Read the model definition and answer for the solid it produces. Units are mm, in the model's axes. Face numbers are marked on the shaded views. A direction names the side the tool comes from. Give positions to 0.01 mm unless a question says otherwise; leave off trailing zeros. Loops run counter-clockwise (first coordinate to the right, second up) from the corner with the lowest first, then second, coordinate; pieces in that order, holes last. Notation, with made-up numbers: (63.5, 23.25) - (113.5, 23.25) arc R26 ccw to (113.5, 43.25) - close; hole circle Ø1 at (45, -32). An arc over 180 degrees is marked (long way). Write item = value, one per line.
```python
from build123d import *

# Parameters (mm, degrees)
SKETCH1_R           = 2
BOSS_EXTRUDE1_DEPTH = 19
SKETCH3_R           = 2
CUT_EXTRUDE2_DEPTH  = 40.953097502
SKETCH4_R           = 4
CUT_EXTRUDE3_DEPTH  = 1.5
CUT_EXTRUDE4_START  = -1.5
SKETCH5_R           = 4
CUT_EXTRUDE4_DEPTH  = 1.5


with BuildPart() as part:
    # Sketch1 → Boss-Extrude1 (new body)
    with BuildSketch(Plane.XY):
        with BuildLine():
            Line((-12.5, -13.5), (12.5, -13.5))
            ThreePointArc((12.5, -13.5), (19.571067812, -10.571067812), (22.5, -3.5))
            Line((22.5, -3.5), (22.5, 3.5))
            ThreePointArc((22.5, 3.5), (19.571067812, 10.571067812), (12.5, 13.5))
            Line((12.5, 13.5), (-12.5, 13.5))
            ThreePointArc((-12.5, 13.5), (-19.571067812, 10.571067812), (-22.5, 3.5))
            Line((-22.5, 3.5), (-22.5, -3.5))
            ThreePointArc((-22.5, -3.5), (-19.571067812, -10.571067812), (-12.5, -13.5))
        make_face()
        with Locations((-18, 0)):
            Circle(SKETCH1_R, mode=Mode.SUBTRACT)
        with Locations((18, 0)):
            Circle(SKETCH1_R, mode=Mode.SUBTRACT)
        with BuildLine():
            Line((-8, -10), (8, -10))
            ThreePointArc((8, -10), (9.414213562, -9.414213562), (10, -8))
            Line((10, -8), (10, 8))
            ThreePointArc((10, 8), (9.414213562, 9.414213562), (8, 10))
            Line((8, 10), (-8, 10))
            ThreePointArc((-8, 10), (-9.414213562, 9.414213562), (-10, 8))
            Line((-10, 8), (-10, -8))
            ThreePointArc((-10, -8), (-9.414213562, -9.414213562), (-8, -10))
        make_face(mode=Mode.SUBTRACT)
    extrude(amount=BOSS_EXTRUDE1_DEPTH)

    # Sketch3 → Cut-Extrude2 (cut, through all)
    with BuildSketch(Plane(origin=(0, 13.5, 0), x_dir=(1, 0, 0), z_dir=(0, 1, 0))):
        with Locations(Location((0, -9.5, 0), (0, 0, 270))):
            Circle(SKETCH3_R)
    extrude(amount=-CUT_EXTRUDE2_DEPTH, mode=Mode.SUBTRACT)

    # Sketch4 → Cut-Extrude3 (cut)
    with BuildSketch(Plane(origin=(0, 13.5, 0), x_dir=(1, 0, 0), z_dir=(0, 1, 0))):
        with Locations(Location((0, -9.5, 0), (0, 0, 270))):
            Circle(SKETCH4_R)
    extrude(amount=-CUT_EXTRUDE3_DEPTH, mode=Mode.SUBTRACT)

    # Sketch5 → Cut-Extrude4 (cut)
    with BuildSketch(Plane.XZ.offset(13.5).offset(CUT_EXTRUDE4_START)):
        with Locations(Location((0, 9.5, 0), (0, 0, 90))):
            Circle(SKETCH5_R)
    extrude(amount=CUT_EXTRUDE4_DEPTH, mode=Mode.SUBTRACT)


solid = part.part
```
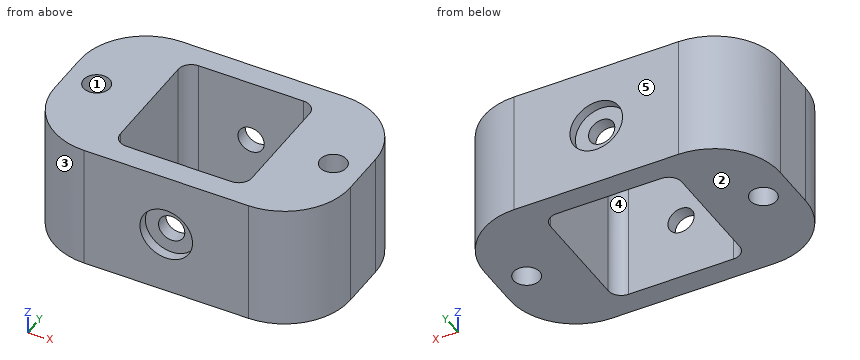
1) A tool of negligible diameter and unlimited length cuts with its end or side. For the marked faces 4 and 5, from which of +Z, -Z, +X, -X, +Y, -Y can it reach the whole face along a straight path? Write none if from no direction.
Output:
face_4 = +Z, -Z
face_5 = +Z, -Z, +X, -X, +Y
2) Each of these flat-tipped pins is pushed along its axis until it touches: P1, Ø2.5, axis at x = 0, z = 8, coming from the +Y side; P2, Ø7, axis at x = 0, z = 9.5, coming from the -Y side; P3, Ø3, axis at x = -16.5, z = 15, coming from the +Y side; P4, Ø2.5, axis at x = 18, y = 0, coming from the +Z side. Where does it stop, or does it pass through?
Output:
P1 = 12
P2 = -12
P3 = 13.18
P4 = through
3) A cutting plane is placed at C-C on x = -7. Determine the outline of the cut face in (y, z).
Output:
outline = (-13.5, 0) - (-10, 0) - (-10, 19) - (-13.5, 19) - close; (10, 0) - (13.5, 0) - (13.5, 19) - (10, 19) - close
4) A cutting plane is placed at B-B on x = 0. Determine the outline of the cut face in (y, z), then the cut area to 3 significant figures.
Output:
outline = (-13.5, 0) - (-10, 0) - (-10, 7.5) - (-12, 7.5) - (-12, 5.5) - (-13.5, 5.5) - close; (-13.5, 13.5) - (-12, 13.5) - (-12, 11.5) - (-10, 11.5) - (-10, 19) - (-13.5, 19) - close; (10, 0) - (13.5, 0) - (13.5, 5.5) - (12, 5.5) - (12, 7.5) - (10, 7.5) - close; (10, 11.5) - (12, 11.5) - (12, 13.5) - (13.5, 13.5) - (13.5, 19) - (10, 19) - close
area = 93.0 mm²
5) Find the intervals of material crossed by probe 1 along Y at (x, z) = (3.5, 5); probe 2 along X at (y, z) = (-2.25, 1); probe 3 along X at (y, z) = (-1.75, 4.25), in increasing order.
Output:
probe_1 = -13.5 to -10, 10 to 13.5
probe_2 = -22.5 to -10, 10 to 22.5
probe_3 = -22.5 to -18.97, -17.03 to -10, 10 to 17.03, 18.97 to 22.5
6) A cutting plane is placed at A-A on z = 9.5. Give the number of separate pieces and of enclosed holes in the cut face, then the cut area to 3 significant figures.
Output:
separate_pieces = 2
enclosed_holes = 2
area = 667 mm²
7) The mould has two halves that part along Y. Classify the marked faces 1, 2 and 3: pulls with the +Y half, pulls with the -Y half, needs draft (parallel to the pull), parting line crosses it, or undercut.
Output:
face_1 = undercut
face_2 = needs draft
face_3 = pulls with the -Y half
8) A cutting plane is placed at D-D on y = 0. Determine the outline of the cut face in (x, z), then the cut area to 3 significant figures.
Output:
outline = (-22.5, 0) - (-20, 0) - (-20, 19) - (-22.5, 19) - close; (-16, 0) - (-10, 0) - (-10, 19) - (-16, 19) - close; (10, 0) - (16, 0) - (16, 19) - (10, 19) - close; (20, 0) - (22.5, 0) - (22.5, 19) - (20, 19) - close
area = 323 mm²
